Input: part model. Units: mm. Frame: model coordinates. Coordinates: 2 decimals unless noted, no trailing zeros. Loops run counter-clockwise (first coordinate to the right, second up) from the corner with the lowest first, then second, coordinate; pieces in that order, holes last.
```python
from build123d import *

# Parameters (mm, degrees)
BOSS_EXTRUDE1_DEPTH = 120


with BuildPart() as part:
    # Sketch1 → Boss-Extrude1 (new body)
    with BuildSketch(Plane(origin=(0, 0, 0), x_dir=(1, 0, 0), z_dir=(0, 1, 0))):
        with BuildLine():
            Line((-105, -30), (-75, -30))
            ThreePointArc((-75, -30), (-45, 0), (-15, -30))
            Line((-15, -30), (15, -30))
            ThreePointArc((15, -30), (45, 0), (75, -30))
            Line((75, -30), (105, -30))
            ThreePointArc((105, -30), (135, 0), (165, -30))
            Line((165, -30), (210, -30))
            Line((210, -30), (210, 30))
            Line((210, 30), (-210, 30))
            Line((-210, 30), (-210, -30))
            Line((-210, -30), (-165, -30))
            ThreePointArc((-165, -30), (-135, 0), (-105, -30))
        make_face()
    extrude(amount=BOSS_EXTRUDE1_DEPTH)


solid = part.part
```
Item 1: Contact query for flat-ended pins moving along their axis: P1, Ø8, axis at x = 128, y = 34, coming from the +Z side; P2, Ø8, axis at x = -135, y = 55.5, coming from the +Z side; P3, Ø5, axis at x = 44.5, y = 61.5, coming from the +Z side. Output: stop coordinate, or through.
Result:
P1: stops at z = 2.09
P2: stops at z = 0.27
P3: stops at z = 0.15
Item 2: Section query A-A (y = 88). Output: boundary loops of the cut face in (x, z), then the cut area to 3 significant figures.
Result:
outline: (-210, -30) - (210, -30) - (210, 30) - (165, 30) arc R30 cw to (105, 30) - (75, 30) arc R30 cw to (15, 30) - (-15, 30) arc R30 cw to (-75, 30) - (-105, 30) arc R30 cw to (-165, 30) - (-210, 30) - close
area: 19,500 mm2
Item 3: Line query: L1, parallel to X at y = 52, z = 16.5; L2, parallel to X at y = 14, z = 21; L3, parallel to Z at x = -145, y = 107. Output: solid intervals per line, ascending.
Result:
L1: x = -210 to -161.79, -108.21 to -71.79, -18.21 to 18.21, 71.79 to 108.21, 161.79 to 210
L2: x = -210 to -163.62, -106.38 to -73.62, -16.38 to 16.38, 73.62 to 106.38, 163.62 to 210
L3: z = -30 to 1.72
Item 4: Section query B-B (x = -27). Output: boundary loops of the cut face in (y, z).
Result:
outline: (0, -30) - (120, -30) - (120, 6) - (0, 6) - close
Item 5: Mould query, pull axis X, two halves, no side actions, for faces 1 (the face through (90, 59, 30)), 2 (the face through (210, 59, 0)), 3 (the face through (44.34, 59.16, 0.007)). Classes: +X half, -X half, draft (parallel to the pull), parting line (faces both ways), or undercut.
Result:
face 1: draft
face 2: +X half
face 3: undercut
Item 6: Section query C-C (x = 45). Output: boundary loops of the cut face in (y, z), then the cut area to 3 significant figures.
Result:
outline: (0, -30) - (120, -30) - (120, 0) - (0, 0) - close
area: 3,600 mm2
